Part model, mm, in its own coordinate system. Face numbers are marked on the shaded views. Give positions to 0.01 mm unless a question says otherwise; leave off trailing zeros. Order: outer loops, then holes, each group sorted by start corner. A loop starts at its lowest first (then second) coordinate and runs counter-clockwise, first axis right, second up. Notation, with made-up numbers: (78, -2) -> (134, -2) arc R5 cw to (134, 4) -> close; hole circle Ø4 at (30, 30.5). An arc over 180 degrees is marked (long way). Write item = value, one per line. Start each with the question number.
Item 1: Band-saw the part on D-D on x = 23. Write the cut outline in (y, z), plus the area to 3 significant figures.
Item 2: Band-saw the part on A-A on z = 8. Write the cut outline in (x, y).
Item 3: Band-saw the part on C-C on z = 35.5. Write the cut outline in (x, y).
Item 4: Drill centre lines: line 1 along X through (y, z) = (3, 68); line 2 along Z through (x, y) = (125.5, 12); line 3 along Y through (x, z) = (120, 1). Where is each one in solid material? Low to high.
Item 5: Pull direction X, two halves, no side cores. Call the marked faces 1, 2 and 3: +X half, -X half, draft (parallel to the pull), parting line (faces both ways), or undercut.
Item 6: Flat gauge pins, fed straight in: P1, Ø1.9, axis at x = 0.5, z = 64.5, coming from the -Y side; P2, Ø1.5, axis at y = -1, z = 9, coming from the +X side; P3, Ø2.5, axis at x = 1, z = 65.5, coming from the +Y side; P4, Ø1.8, axis at y = 4.5, z = 67.6, coming from the -X side. Where does each tip first touch, or does it go through?
Item 7: Band-saw the part on B-B on x = 139.5. Write the cut outline in (y, z), plus the area to 3 significant figures.
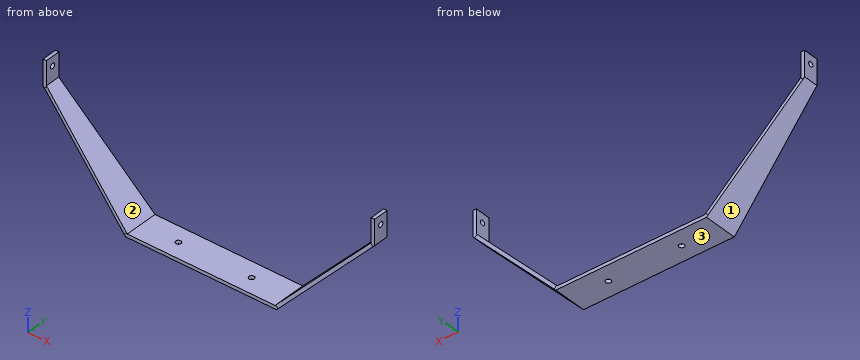
```python
from build123d import *

# Parameters (mm, degrees)
SKETCH_1_W          = 2
SKETCH_1_H          = 15
EXTRUDE_1_DEPTH     = 9
EXTRUDE_1_2_DEPTH   = 9
SKETCH_2_R          = 1.5
CUT_EXTRUDE_1_DEPTH = 212.220264179
SKETCH_3_W          = 90
SKETCH_3_H          = 20
EXTRUDE_2_DEPTH     = 2
SKETCH_4_W          = 1.362837056
SKETCH_4_H          = 9
SKETCH_4_W_2        = 1.463787949
SKETCH_4_H_2        = 20
EXTRUDE_3_DEPTH     = 2
SKETCH_6_R          = 1.6
CUT_EXTRUDE_2_DEPTH = 10


with BuildPart() as part:
    # Sketch 1 → Extrude 1 (new body)
    with BuildSketch(Plane(origin=(0, 0, 0), x_dir=(1, 0, 0), z_dir=(0, 1, 0))):
        with Locations((1, -65.5)):
            Rectangle(SKETCH_1_W, SKETCH_1_H)
    extrude(amount=EXTRUDE_1_DEPTH)


with BuildPart() as body_2:
    # Sketch 1 → Extrude 1 2 (new body)
    with BuildSketch(Plane(origin=(0, 0, 0), x_dir=(1, 0, 0), z_dir=(0, 1, 0))):
        with Locations((197, -65.5)):
            Rectangle(SKETCH_1_W, SKETCH_1_H)
    extrude(amount=EXTRUDE_1_2_DEPTH)


with BuildPart() as cut_extrude_1_tool:
    # Sketch 2 → Cut-Extrude 1 (new, through all)
    with BuildSketch(Plane(origin=(198, 0, 0), x_dir=(0, 0, -1), z_dir=(1, 0, 0))):
        with Locations((-67.601305665, 4.5)):
            Circle(SKETCH_2_R)
    extrude(amount=-CUT_EXTRUDE_1_DEPTH)


with BuildPart() as part_1:
    add(part.part)

    # Cut-Extrude 1: cut by cut_extrude_1_tool
    add(cut_extrude_1_tool.part, mode=Mode.SUBTRACT)


with BuildPart() as body_2_1:
    add(body_2.part)

    # Cut-Extrude 1: cut by cut_extrude_1_tool
    add(cut_extrude_1_tool.part, mode=Mode.SUBTRACT)



with BuildPart() as body_3:
    # Sketch 3 → Extrude 2 (new body)
    with BuildSketch(Plane.XY):
        with Locations((99, 4.5)):
            Rectangle(SKETCH_3_W, SKETCH_3_H)
    extrude(amount=EXTRUDE_2_DEPTH)


with BuildPart() as body_2_2:
    add(body_2_1.part)

    add(body_3.part)  # Extrude 3 merges body 3
    # Sketch 4 → Extrude 3 (add)
    with BuildSketch(Plane(origin=(77.136305732, 0, -71.81656051), x_dir=(-0.6814185279188432, 0, -0.7318939744313494), z_dir=(0.7318939744313494, 0, -0.6814185279188432))):
        with Locations((-176.689300517, 4.5)):
            Rectangle(SKETCH_4_W, SKETCH_4_H)
        Polygon((-176.007881989, 9), (-99.588055969, 14.5), (-99.588055969, -5.5), (-176.007881989, 0), align=None)
        with Locations((-98.856161995, 4.5)):
            Rectangle(SKETCH_4_W_2, SKETCH_4_H_2)
    extrude_3 = extrude(amount=-EXTRUDE_3_DEPTH)

    # Mirror 1: Extrude 3 across plane
    add(extrude_3.mirror(Plane(origin=(99, 0, 0), x_dir=(0, 0, 1), z_dir=(1, 0, 0))))

    # Combine 1: union part
    add(part_1.part)

    # Sketch 6 → Cut-Extrude 2 (cut)
    with BuildSketch(Plane(origin=(0, 0, 0), x_dir=(-1, 0, 0), z_dir=(0, 0, -1))):
        with Locations((-120.9, 4.5)):
            Circle(SKETCH_6_R)
        with Locations((-77.1, 4.5)):
            Circle(SKETCH_6_R)
    extrude(amount=-CUT_EXTRUDE_2_DEPTH, mode=Mode.SUBTRACT)


solid = body_2_2.part
```
Values found:
q1.outline = (-2.33, 33.3) -> (11.33, 33.3) -> (11.18, 36.23) -> (-2.18, 36.23) -> close
q1.area = 39.6 mm^2
q2.outline = (46.55, -4.82) -> (49.28, -4.95) -> (49.28, 13.95) -> (46.55, 13.82) -> close; (148.72, -4.95) -> (151.45, -4.82) -> (151.45, 13.82) -> (148.72, 13.95) -> close
q3.outline = (20.95, -2.11) -> (23.68, -2.25) -> (23.68, 11.25) -> (20.95, 11.11) -> close; (174.32, -2.25) -> (177.05, -2.11) -> (177.05, 11.11) -> (174.32, 11.25) -> close
q4.line_1 = 0 to 2, 196 to 198
q4.line_2 = 0 to 2
q4.line_3 = -5.5 to 3.18, 5.82 to 14.5
q5.face_1 = -X half
q5.face_2 = undercut
q5.face_3 = draft
q6.P1 = 0
q6.P2 = 153.08
q6.P3 = 9
q6.P4 = through
q7.outline = (-5.5, 0) -> (14.5, 0) -> (14.5, 2) -> (-5.5, 2) -> close
q7.area = 40.0 mm^2
